Verification items for this drawing (mm, ordinates from the low corner). A direction names the side the tool comes from. Give positions to 0.01 mm unless a question says otherwise; leave off trailing zeros. Order: outer loops, then holes, each group sorted by start corner. A loop starts at its lowest first (then second) coordinate and runs counter-clockwise, first axis right, second up.
(1) Mould release check, pull along Y, two halves, no side actions. Record for the marked faces 1, 2 and 3: pulls with the +Y half, pulls with the -Y half, needs draft (parallel to the pull), parting line crosses it, or undercut.
(2) Scan lines: L1, parallel to Y at x = 116.5, z = 40; L2, parallel to Y at x = 10, z = 28; L3, parallel to Z at x = 139.5, y = 25. Record each from-to range of solid material in increasing order.
(3) Sectioned sample at A-A on x = 124.5. Record the cut outline in (y, z), plus the area to 3 significant figures.
(4) Sectioned sample at B-B on y = 15. Record the cut outline in (x, z).
(5) Sectioned sample at C-C on z = 4. Record the cut outline in (x, y), plus the area to 3 significant figures.
(6) Access from +Z, -Z, +X, -X, +Y, -Y to the whole of each face (thin tool, end or side, straight path). Record for the marked faces 4, 5 and 6.
(7) Sectioned sample at D-D on y = 29.5. Record the cut outline in (x, z).
(8) Gauge pin test, flat ends, axial feed: pin 1 (15 mm diameter, centred on x = 102.5, y = 49, fed in from +Z); pin 2 (10 mm diameter, centred on x = 99, y = 20.5, fed in from -Z). Record the tip position at first contact, or that the pin passes through.
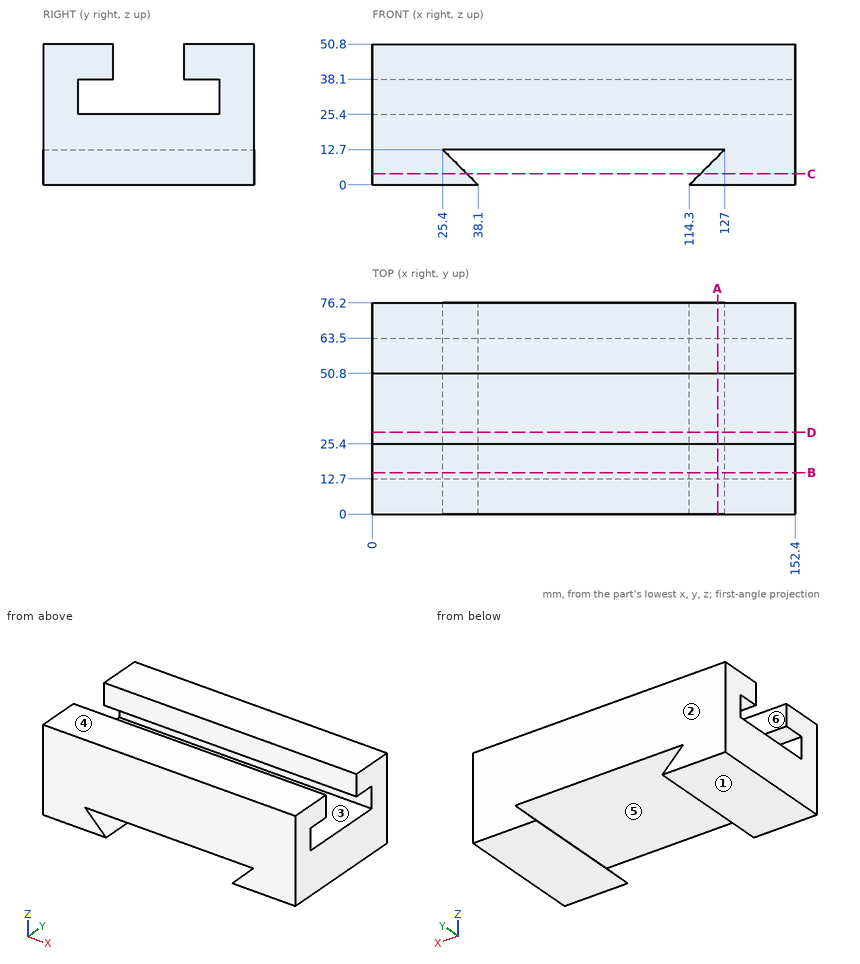
Ans:
1. face 1: needs draft
1. face 2: pulls with the +Y half
1. face 3: undercut
2. L1: y = 0 to 25.4, 50.8 to 76.2
2. L2: y = 0 to 12.7, 63.5 to 76.2
2. L3: z = 0 to 25.4, 38.1 to 50.8
3. outline: (0, 0) - (76.2, 0) - (76.2, 10.2) - (0, 10.2) - close; (0, 12.7) - (76.2, 12.7) - (76.2, 50.8) - (50.8, 50.8) - (50.8, 38.1) - (63.5, 38.1) - (63.5, 25.4) - (12.7, 25.4) - (12.7, 38.1) - (25.4, 38.1) - (25.4, 50.8) - (0, 50.8) - close
3. area: 2,710 mm2
4. outline: (0, 0) - (38.1, 0) - (25.4, 12.7) - (127, 12.7) - (114.3, 0) - (152.4, 0) - (152.4, 25.4) - (0, 25.4) - close; (0, 38.1) - (152.4, 38.1) - (152.4, 50.8) - (0, 50.8) - close
5. outline: (0, 0) - (34.1, 0) - (34.1, 76.2) - (0, 76.2) - close; (118.3, 0) - (152.4, 0) - (152.4, 76.2) - (118.3, 76.2) - close
5. area: 5,200 mm2
6. face 4: +Z, +X, -X, +Y, -Y
6. face 5: +Y, -Y
6. face 6: +Z, +X, -X
7. outline: (0, 0) - (38.1, 0) - (25.4, 12.7) - (127, 12.7) - (114.3, 0) - (152.4, 0) - (152.4, 25.4) - (0, 25.4) - close
8. pin 1: stops at z = 50.8
8. pin 2: stops at z = 12.7
